Part model, mm, in its own coordinate system. Face numbers are marked on the shaded views. Give positions to 0.01 mm unless a question says otherwise; leave off trailing zeros. Order: outer loops, then holes, each group sorted by start corner. A loop starts at its lowest first (then second) coordinate and runs counter-clockwise, first axis right, second up.
1. Slice it at B-B on z = 273.05. List the corners of the cut face in (x, y) (3 decimals).
2. Slice it at A-A on y = 21.5. List the corners of the cut face in (x, z) (3 decimals), and give its area (3 significant figures).
3. Probe line 1 (X direction, y = 6.75, z = 99) (3 decimals); line 2 (X direction, y = 1.15, z = 241.3) (3 decimals); line 3 (Y direction, x = 7.5, z = 91.5) (3 decimals). List the from-to ranges inside material, lowest first.
4. Mould opens along X. For the marked faces 1 and 2 say: +X half, -X half, draft (parallel to the pull), parting line (faces both ways), or undercut.
5. Slice it at D-D on z = 437. List the corners of the cut face in (x, y) (3 decimals), and give its area (3 significant figures).
6. Slice it at C-C on x = 10. List the corners of the cut face in (y, z) (3 decimals).
7. Drop a flat-ended pin along its axis: pin 1 Ø13.5 at (x, z) = (26, 137) entering from +Y (3 decimals). Give the stop position or say it passes through.
from build123d import *

# Parameters (mm, degrees)
BOSS_EXTRUDE1_DEPTH = 508
CUT_EXTRUDE1_REACH  = 5.175
SKETCH2_R           = 14.2875


with BuildPart() as part:
    # Sketch1 → Boss-Extrude1 (new body)
    with BuildSketch(Plane.XY):
        Polygon((47.625, 3.175), (47.625, 25.4), (50.8, 25.4), (50.8, 0), (0, 0), (0, 25.4), (3.175, 25.4), (3.175, 3.175), align=None)
    extrude(amount=BOSS_EXTRUDE1_DEPTH)

    # Sketch2 → Cut-Extrude1 (cut, up to next)
    with BuildSketch(Plane(origin=(0, 3.175, 0), x_dir=(1, 0, 0), z_dir=(0, 1, 0)), mode=Mode.PRIVATE) as cut_extrude1_sk1:
        with Locations((18.7325, -336.55)):
            Circle(SKETCH2_R)
    cut_extrude1_tool1 = extrude(cut_extrude1_sk1.sketch, amount=-CUT_EXTRUDE1_REACH, mode=Mode.PRIVATE) & part.part
    add(cut_extrude1_tool1.solids().sort_by_distance((18.7325, 3.175, 336.55))[0], mode=Mode.SUBTRACT)
    # Sketch2 → Cut-Extrude1 (cut, up to next)
    with BuildSketch(Plane(origin=(0, 3.175, 0), x_dir=(1, 0, 0), z_dir=(0, 1, 0)), mode=Mode.PRIVATE) as cut_extrude1_sk2:
        with Locations((32.0675, -304.8)):
            Circle(SKETCH2_R)
    cut_extrude1_tool2 = extrude(cut_extrude1_sk2.sketch, amount=-CUT_EXTRUDE1_REACH, mode=Mode.PRIVATE) & part.part
    add(cut_extrude1_tool2.solids().sort_by_distance((32.0675, 3.175, 304.8))[0], mode=Mode.SUBTRACT)
    # Sketch2 → Cut-Extrude1 (cut, up to next)
    with BuildSketch(Plane(origin=(0, 3.175, 0), x_dir=(1, 0, 0), z_dir=(0, 1, 0)), mode=Mode.PRIVATE) as cut_extrude1_sk3:
        with Locations((18.7325, -273.05)):
            Circle(SKETCH2_R)
    cut_extrude1_tool3 = extrude(cut_extrude1_sk3.sketch, amount=-CUT_EXTRUDE1_REACH, mode=Mode.PRIVATE) & part.part
    add(cut_extrude1_tool3.solids().sort_by_distance((18.7325, 3.175, 273.05))[0], mode=Mode.SUBTRACT)
    # Sketch2 → Cut-Extrude1 (cut, up to next)
    with BuildSketch(Plane(origin=(0, 3.175, 0), x_dir=(1, 0, 0), z_dir=(0, 1, 0)), mode=Mode.PRIVATE) as cut_extrude1_sk4:
        with Locations((32.0675, -241.3)):
            Circle(SKETCH2_R)
    cut_extrude1_tool4 = extrude(cut_extrude1_sk4.sketch, amount=-CUT_EXTRUDE1_REACH, mode=Mode.PRIVATE) & part.part
    add(cut_extrude1_tool4.solids().sort_by_distance((32.0675, 3.175, 241.3))[0], mode=Mode.SUBTRACT)
    # Sketch2 → Cut-Extrude1 (cut, up to next)
    with BuildSketch(Plane(origin=(0, 3.175, 0), x_dir=(1, 0, 0), z_dir=(0, 1, 0)), mode=Mode.PRIVATE) as cut_extrude1_sk5:
        with Locations((18.7325, -209.55)):
            Circle(SKETCH2_R)
    cut_extrude1_tool5 = extrude(cut_extrude1_sk5.sketch, amount=-CUT_EXTRUDE1_REACH, mode=Mode.PRIVATE) & part.part
    add(cut_extrude1_tool5.solids().sort_by_distance((18.7325, 3.175, 209.55))[0], mode=Mode.SUBTRACT)
    # Sketch2 → Cut-Extrude1 (cut, up to next)
    with BuildSketch(Plane(origin=(0, 3.175, 0), x_dir=(1, 0, 0), z_dir=(0, 1, 0)), mode=Mode.PRIVATE) as cut_extrude1_sk6:
        with Locations((32.0675, -177.8)):
            Circle(SKETCH2_R)
    cut_extrude1_tool6 = extrude(cut_extrude1_sk6.sketch, amount=-CUT_EXTRUDE1_REACH, mode=Mode.PRIVATE) & part.part
    add(cut_extrude1_tool6.solids().sort_by_distance((32.0675, 3.175, 177.8))[0], mode=Mode.SUBTRACT)


solid = part.part
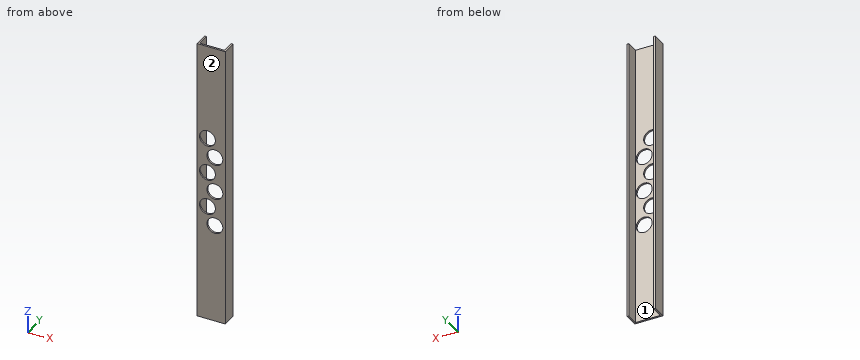
Data:
1. outline: (0, 0) - (4.445, 0) - (4.445, 3.175) - (3.175, 3.175) - (3.175, 25.4) - (0, 25.4) - close; (33.02, 0) - (50.8, 0) - (50.8, 25.4) - (47.625, 25.4) - (47.625, 3.175) - (33.02, 3.175) - close
2. outline: (0, 0) - (3.175, 0) - (3.175, 508) - (0, 508) - close; (47.625, 0) - (50.8, 0) - (50.8, 508) - (47.625, 508) - close
2. area: 3,230 mm2
3. line 1: x = 0 to 3.175, 47.625 to 50.8
3. line 2: x = 0 to 17.78, 46.355 to 50.8
3. line 3: y = 0 to 3.175
4. face 1: undercut
4. face 2: draft
5. outline: (0, 0) - (50.8, 0) - (50.8, 25.4) - (47.625, 25.4) - (47.625, 3.175) - (3.175, 3.175) - (3.175, 25.4) - (0, 25.4) - close
5. area: 302 mm2
6. outline: (0, 0) - (3.175, 0) - (3.175, 198.242) - (0, 198.242) - close; (0, 220.858) - (3.175, 220.858) - (3.175, 261.742) - (0, 261.742) - close; (0, 284.358) - (3.175, 284.358) - (3.175, 325.242) - (0, 325.242) - close; (0, 347.858) - (3.175, 347.858) - (3.175, 508) - (0, 508) - close
7. pin 1: stops at y = 3.175
